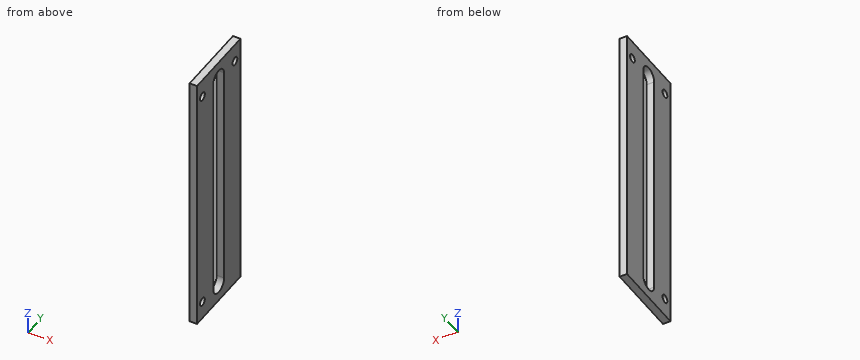
Solid Edge part; units mm, degrees
sketch "Sketch1" plane through (-15, 0, 0) normal (1, 0, 0) x (0, 1, 0)
  circle A0 centre (69.5, 286) radius 1.1
  line L0 (79.5, 223.5) -> (79.5, 286)
  line L1 (74.5, 286) -> (74.5, 223.5)
  arc A1 (74.5, 286) -> (79.5, 286) centre (77, 286) cw
  arc A2 (79.5, 223.5) -> (74.5, 223.5) centre (77, 223.5) cw
  line L2 (87, 291) -> (67, 291)
  line L3 (67, 291) -> (67, 218.5)
  line L4 (67, 218.5) -> (87, 218.5)
  line L5 (87, 218.5) -> (87, 291)
  circle A3 centre (84.5, 286) radius 1.1
  circle A4 centre (69.5, 223.5) radius 1.1
extrude "Protrusion1" add sketch "Sketch1" along normal blind 2
For this review, take the finished solid that the model builds, in its own axes (mm). Give positions to 0.01 mm unless a question says otherwise; leave off trailing zeros. Write each loop counter-clockwise with the first axis right and the second up, starting at its lowest first coordinate (ties: lowest second). Pieces come first, ordered by that corner, then holes. Notation, with made-up numbers: M -31.5,64 L -20.5,64 A29 cw -20.5,86 Z; hole C 1,80 d3. An arc over 180 degrees is marked long. Answer as a JSON object with one key per item and string values. Group by question number.
Item 1: Consider section A-A on y = 77. Write out the cut boundary in (x, z).
Item 2: For pin 1 Ø1.5 at (y, z) = (78, 283) entering from +X, flat-tipped, find the tip position at first contact; note if it passes through.
Item 3: Consider section C-C on y = 69.5. Write out the cut boundary in (x, z).
Item 4: For probe 1 along Y at (x, z) = (-14.55, 223.5); probe 2 along Z at (x, y) = (-13.9, 69.5); probe 3 along Y at (x, z) = (-13.7, 286), list the stretches that pass through material, from the lowest coordinate up. Write a range as [from, to].
Item 5: Consider section D-D on x = -13.8. Write out the cut boundary in (y, z).
Item 6: Consider section B-B on z = 273. Write out the cut boundary in (x, y), plus the area to 3 significant figures.
Check result:
{
 "1": {"outline": "M -15,218.5 L -13,218.5 L -13,221 L -15,221 Z; M -15,288.5 L -13,288.5 L -13,291 L -15,291 Z"},
 "2": {"pin 1": "passes through"},
 "3": {"outline": "M -15,218.5 L -13,218.5 L -13,222.4 L -15,222.4 Z; M -15,224.6 L -13,224.6 L -13,284.9 L -15,284.9 Z; M -15,287.1 L -13,287.1 L -13,291 L -15,291 Z"},
 "4": {"probe 1": "y = [67, 68.4], [70.6, 74.5], [79.5, 87]", "probe 2": "z = [218.5, 222.4], [224.6, 284.9], [287.1, 291]", "probe 3": "y = [67, 68.4], [70.6, 74.5], [79.5, 83.4], [85.6, 87]"},
 "5": {"outline": "M 67,218.5 L 87,218.5 L 87,291 L 67,291 Z; hole C 69.5,223.5 d2.2; hole C 69.5,286 d2.2; hole M 74.5,223.5 A2.5 ccw 79.5,223.5 L 79.5,286 A2.5 ccw 74.5,286 Z; hole C 84.5,286 d2.2"},
 "6": {"outline": "M -15,67 L -13,67 L -13,74.5 L -15,74.5 Z; M -15,79.5 L -13,79.5 L -13,87 L -15,87 Z", "area": "30.0 mm^2"}
}
